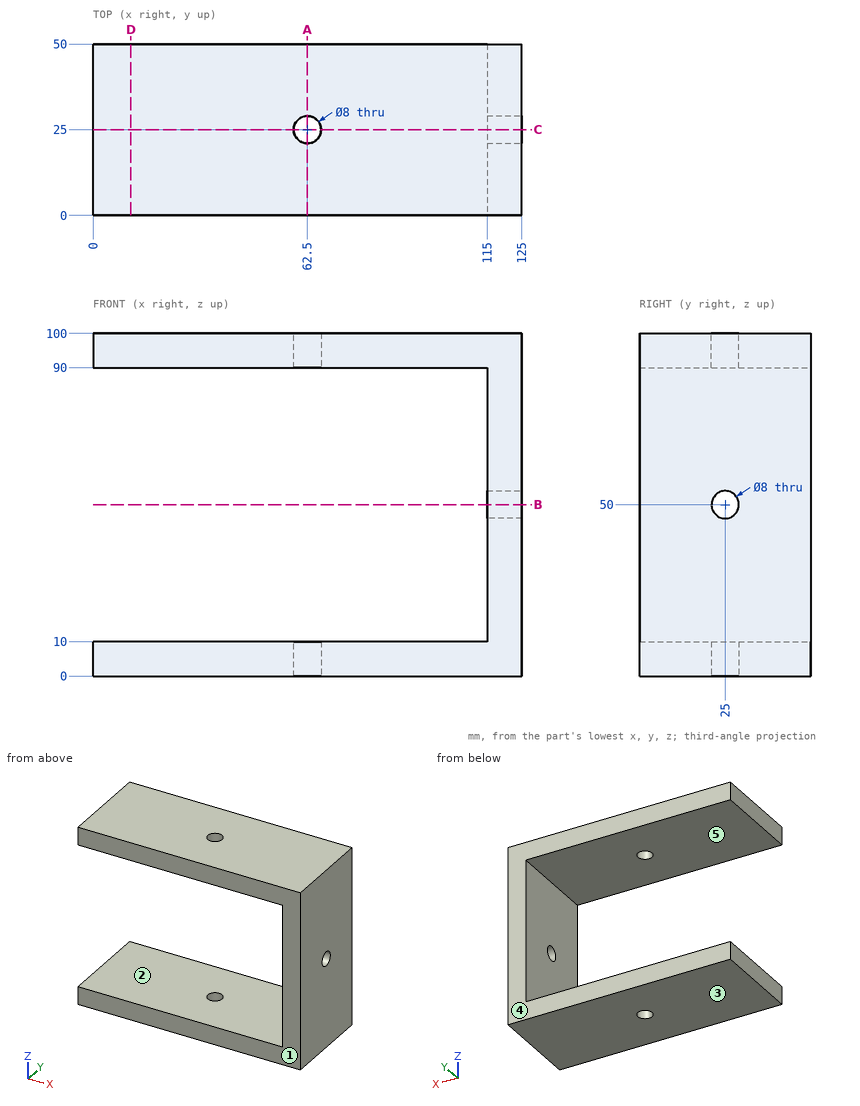
Print and shaded views of the part. All mm, measured from the part's lowest x, y and z. A direction names the side the tool comes from. Coordinates: 2 decimals unless noted, no trailing zeros. Loops run counter-clockwise (first coordinate to the right, second up) from the corner with the lowest first, then second, coordinate; pieces in that order, holes last. Notation, with made-up numbers: (16.25, 65) - (30.25, 65) arc R18 ccw to (30.25, 92) - close; hole circle Ø2 at (51, 60.25). An arc over 180 degrees is marked (long way). Write item = value, one per line. Start each with the question number.
Item 1: Cut at D-D, the plane x = 11. Give the cut face in (y, z), and give its area (3 significant figures).
Item 2: Cut at A-A, the plane x = 62.5. Give the cut face in (y, z), and give its area (3 significant figures).
Item 3: Wall check: L1, parallel to Z at x = 105, y = 32.5; L2, parallel to Y at x = 62.5, z = 98.25; L3, parallel to X at y = 9, z = 44.5. Give the ranges that are in metal, low to high. Write a range as from..to.
Item 4: Flat gauge pin, fed straight in: pin 1 Ø1.5 at (y, z) = (27, 20) entering from -X. Where does the tip first touch, or does it go through?
Item 5: 3-axis set-ups, long thin cutter, end or side, ignore diameter. For the marked faces 1 and 2: which of +Z, -Z, +X, -X, +Y, -Y reach the whole face in a straight line?
Item 6: Mould opens along Z. For the marked faces 3, 4 and 5 say: released by +Z, released by -Z, zero draft, split by the parting line, or undercut.
Item 7: Cut at C-C, the plane y = 25. Give the cut face in (x, z), and give its area (3 significant figures).
Item 8: Cut at B-B, the plane z = 50. Give the cut face in (x, y), and give its area (3 significant figures).
The answers:
q1.outline = (0, 0) - (50, 0) - (50, 10) - (0, 10) - close; (0, 90) - (50, 90) - (50, 100) - (0, 100) - close
q1.area = 1,000 mm2
q2.outline = (0, 0) - (21, 0) - (21, 10) - (0, 10) - close; (0, 90) - (21, 90) - (21, 100) - (0, 100) - close; (29, 0) - (50, 0) - (50, 10) - (29, 10) - close; (29, 90) - (50, 90) - (50, 100) - (29, 100) - close
q2.area = 840 mm2
q3.L1 = 0..10, 90..100
q3.L2 = 0..21, 29..50
q3.L3 = 115..125
q4.pin_1 = 115
q5.face_1 = +Z, -Z, +X, -X, -Y
q5.face_2 = -X, +Y, -Y
q6.face_3 = released by -Z
q6.face_4 = zero draft
q6.face_5 = undercut
q7.outline = (0, 0) - (58.5, 0) - (58.5, 10) - (0, 10) - close; (0, 90) - (58.5, 90) - (58.5, 100) - (0, 100) - close; (66.5, 0) - (125, 0) - (125, 46) - (115, 46) - (115, 10) - (66.5, 10) - close; (66.5, 90) - (115, 90) - (115, 54) - (125, 54) - (125, 100) - (66.5, 100) - close
q7.area = 3,060 mm2
q8.outline = (115, 0) - (125, 0) - (125, 21) - (115, 21) - close; (115, 29) - (125, 29) - (125, 50) - (115, 50) - close
q8.area = 420 mm2
